Source: CAD feature listing. Evaluate the final solid. Frame: model axes, mm. Coordinates: 2 decimals unless noted, no trailing zeros. Write each loop counter-clockwise with the first axis right and the second up, starting at its lowest first coordinate (ties: lowest second). Pieces come first, ordered by that corner, then holes. Notation, with made-up numbers: M 83,35 L 87,35 A29 cw 87,57 Z; hole C 80.25,34.5 d3. An arc over 180 degrees is marked long. Write item = value, one per line. Start each with the question number.
1. Section query D-D (z = 5). Give the number of separate pieces and of enclosed holes in the cut face, then the cut area to 3 significant figures.
2. Section query B-B (y = -10.5). Output: boundary loops of the cut face in (x, z), then the cut area to 3 significant figures.
3. Pull-direction query (X, two-part tool) for faces 1 (the face through (180, -1, 6)), 2 (the face through (137.86, 34.9, 6.08)), 3 (the face through (-3, 9, 0)), 4 (the face through (-180, -1, 6)); classes: pulls with the +X half, pulls with the -X half, needs draft (parallel to the pull), parting line crosses it, or undercut.
4. Section query C-C (x = 5). Output: boundary loops of the cut face in (y, z).
5. Line query: line 1 along Y through (x, z) = (23.5, 5.5); line 2 along Y through (x, z) = (45, 7.5); line 3 along X through (y, z) = (-10, 10.25). Output: solid intervals per line, ascending.
6. Section query A-A (y = 34). Output: boundary loops of the cut face in (x, z).
7. Pin query (flat end, axial travel): pin 1 Ø9.5 at (x, y) = (-45, 34) entering from +Z. Return the tip coordinate at first contact, or that it passes through.
```python
from build123d import *

# Parameters (mm, degrees)
SKETCH1_W           = 360
SKETCH1_H           = 80
BOSS_EXTRUDE1_DEPTH = 12
CUT_EXTRUDE1_REACH  = 186.781
SKETCH2_R           = 3
LPATTERN1_COUNT     = 4
LPATTERN1_PITCH     = 90
CUT_EXTRUDE2_REACH  = 186.781
SKETCH3_R           = 13
CUT_EXTRUDE3_REACH  = 186.781
SKETCH4_R           = 2


with BuildPart() as part:
    # Sketch1 → Boss-Extrude1 (new body)
    with BuildSketch(Plane.XY):
        Rectangle(SKETCH1_W, SKETCH1_H)
    extrude(amount=BOSS_EXTRUDE1_DEPTH)

    # Sketch2 → Cut-Extrude1 (cut, up to next)
    with BuildSketch(Plane.XY.offset(12), mode=Mode.PRIVATE) as cut_extrude1_sk1:
        with Locations((135, 34)):
            Circle(SKETCH2_R)
    cut_extrude1_tool1 = extrude(cut_extrude1_sk1.sketch, amount=-CUT_EXTRUDE1_REACH, mode=Mode.PRIVATE) & part.part
    cut_extrude1 = cut_extrude1_tool1.solids().sort_by_distance((135, 34, 12))[0]
    add(cut_extrude1, mode=Mode.SUBTRACT)

    # LPattern1: Cut-Extrude1 ×4
    with Locations(*[(-i * LPATTERN1_PITCH, 0, 0) for i in range(1, LPATTERN1_COUNT)]):
        add(cut_extrude1, mode=Mode.SUBTRACT)

    # Sketch3 → Cut-Extrude2 (cut, up to next)
    with BuildSketch(Plane.XY.offset(12), mode=Mode.PRIVATE) as cut_extrude2_sk1:
        with Locations((0, -10.5)):
            Circle(SKETCH3_R)
    cut_extrude2_tool1 = extrude(cut_extrude2_sk1.sketch, amount=-CUT_EXTRUDE2_REACH, mode=Mode.PRIVATE) & part.part
    add(cut_extrude2_tool1.solids().sort_by_distance((0, -10.5, 12))[0], mode=Mode.SUBTRACT)

    # Sketch4 → Cut-Extrude3 (cut, up to next)
    with BuildSketch(Plane.XY.offset(12), mode=Mode.PRIVATE) as cut_extrude3_sk1:
        with Locations((-23.5, 13)):
            Circle(SKETCH4_R)
    cut_extrude3_tool1 = extrude(cut_extrude3_sk1.sketch, amount=-CUT_EXTRUDE3_REACH, mode=Mode.PRIVATE) & part.part
    # Sketch4 → Cut-Extrude3 (cut, up to next)
    with BuildSketch(Plane.XY.offset(12), mode=Mode.PRIVATE) as cut_extrude3_sk2:
        with Locations((-23.5, -34)):
            Circle(SKETCH4_R)
    cut_extrude3_tool2 = extrude(cut_extrude3_sk2.sketch, amount=-CUT_EXTRUDE3_REACH, mode=Mode.PRIVATE) & part.part
    cut_extrude3_1 = cut_extrude3_tool1.solids().sort_by_distance((-23.5, 13, 12))[0]
    add(cut_extrude3_1, mode=Mode.SUBTRACT)
    cut_extrude3_2 = cut_extrude3_tool2.solids().sort_by_distance((-23.5, -34, 12))[0]
    add(cut_extrude3_2, mode=Mode.SUBTRACT)
    cut_extrude3 = cut_extrude3_1 + cut_extrude3_2  # Cut-Extrude3 as one shape, for the pattern or mirror that repeats it

    # Mirror2: Cut-Extrude3 across plane
    add(cut_extrude3.mirror(Plane(origin=(0, 0, 0), x_dir=(0, 0, 1), z_dir=(1, 0, 0))), mode=Mode.SUBTRACT)


solid = part.part
```
Results are:
q1.separate_pieces = 1
q1.enclosed_holes = 9
q1.area = 28,100 mm^2
q2.outline = M -180,0 L -13,0 L -13,12 L -180,12 Z; M 13,0 L 180,0 L 180,12 L 13,12 Z
q2.area = 4,010 mm^2
q3.face_1 = pulls with the +X half
q3.face_2 = undercut
q3.face_3 = needs draft
q3.face_4 = pulls with the -X half
q4.outline = M -40,0 L -22.5,0 L -22.5,12 L -40,12 Z; M 1.5,0 L 40,0 L 40,12 L 1.5,12 Z
q5.line_1 = -40 to -36, -32 to 11, 15 to 40
q5.line_2 = -40 to 31, 37 to 40
q5.line_3 = -180 to -12.99, 12.99 to 180
q6.outline = M -180,0 L -138,0 L -138,12 L -180,12 Z; M -132,0 L -48,0 L -48,12 L -132,12 Z; M -42,0 L 42,0 L 42,12 L -42,12 Z; M 48,0 L 132,0 L 132,12 L 48,12 Z; M 138,0 L 180,0 L 180,12 L 138,12 Z
q7.pin_1 = 12
